from build123d import *

# Parameters (mm, degrees)
SKETCH1_W           = 22
SKETCH1_H           = 63.25
BOSS_EXTRUDE1_DEPTH = 17.4
SKETCH2_W           = 10.1
SKETCH2_H           = 7.15
CUT_EXTRUDE1_DEPTH  = 8.4
SKETCH3_R           = 2.325
CUT_EXTRUDE2_DEPTH  = 38.734607789


with BuildPart() as part:
    # Sketch1 → Boss-Extrude1 (new body)
    with BuildSketch(Plane(origin=(0, 0, 0), x_dir=(1, 0, 0), z_dir=(0, 1, 0))):
        Rectangle(SKETCH1_W, SKETCH1_H)
    extrude(amount=BOSS_EXTRUDE1_DEPTH)

    # Sketch2 → Cut-Extrude1 (cut)
    with BuildSketch(Plane(origin=(0, 17.4, 0), x_dir=(1, 0, 0), z_dir=(0, 1, 0))):
        with Locations((-5.95, 18.05)):
            Rectangle(SKETCH2_W, SKETCH2_H)
        with Locations((5.95, 18.05)):
            Rectangle(SKETCH2_W, SKETCH2_H)
        with Locations((-5.95, 9.025)):
            Rectangle(SKETCH2_W, SKETCH2_H)
        with Locations((5.95, 9.025)):
            Rectangle(SKETCH2_W, SKETCH2_H)
        with Locations((-5.95, 0)):
            Rectangle(SKETCH2_W, SKETCH2_H)
        with Locations((5.95, 0)):
            Rectangle(SKETCH2_W, SKETCH2_H)
        with Locations((-5.95, -9.025)):
            Rectangle(SKETCH2_W, SKETCH2_H)
        with Locations((5.95, -9.025)):
            Rectangle(SKETCH2_W, SKETCH2_H)
        with Locations((-5.95, -18.05)):
            Rectangle(SKETCH2_W, SKETCH2_H)
        with Locations((5.95, -18.05)):
            Rectangle(SKETCH2_W, SKETCH2_H)
    extrude(amount=-CUT_EXTRUDE1_DEPTH, mode=Mode.SUBTRACT)

    # Sketch3 → Cut-Extrude2 (cut, through all)
    with BuildSketch(Plane(origin=(0, 0, 0), x_dir=(1, 0, 0), z_dir=(0, 1, 0))):
        with Locations(Location((0, 26.675, 0), (0, 0, 270))):
            Circle(SKETCH3_R)
        with Locations(Location((0, -26.675, 0), (0, 0, 270))):
            Circle(SKETCH3_R)
    extrude(amount=CUT_EXTRUDE2_DEPTH, mode=Mode.SUBTRACT)


solid = part.part
Could you check a few things on this model? Use its own coordinates, in mm. A direction names the side the tool comes from. Coordinates: 2 decimals unless noted, no trailing zeros. Write each loop counter-clockwise with the first axis right and the second up, starting at its lowest first coordinate (ties: lowest second). Pieces come first, ordered by that corner, then holes. Notation, with made-up numbers: (46.5, -38.5) - (92.5, -38.5) arc R18 ccw to (92.5, -22.5) - close; hole circle Ø2 at (45.25, 1). An arc over 180 degrees is marked (long way). Put each result on its own line as item: value. Start each with the question number.
Q1. Which directions (+Z, -Z, +X, -X, +Y, -Y) give clear straight access to the entire face, cutting with the end or side of a thin tool? Please do faces 1 (the flat face through (0.9, 13, -9)), 2 (the cylindrical face through (0.698, 8.578, -24.457)), 3 (the flat face through (-0.9, 13, 0)).
Q2. Please list where these lines run through material, in increasing order: L1, parallel to Z at x = 0, y = 4.5 (3 decimals); L2, parallel to Z at x = -8.25, y = 15 (3 decimals); L3, parallel to Z at x = -0.5, y = 7.25 (3 decimals).
Q3. I want a section at D-D on y = 14.25. Count the separate pieces of the cut face and the enclosed holes in it, plus the area to 3 significant figures.
Q4. I'm going to push flat-ended pins straight in: P1, Ø2, axis at x = -5, z = 7.5, coming from the +Y side; P2, Ø4, axis at x = 0.5, z = 23.5, coming from the -Y side; P3, Ø2, axis at y = 14.5, z = 10.5, coming from the -X side. Where does each tip first touch, or does it pass through?
Q5. Thinking about a two-plate mould opening in Z: for faces 4 (the flat face through (11, 7, 0)), 5 (the flat face through (-0.9, 13, -18)), 6 (the cylindrical face through (1.57, 8.58, 24.96)), which applies, pulls with the +Z half, pulls with the -Z half, needs draft (parallel to the pull), parting line crosses it, or undercut?
Q6. I want a section at A-A on x = 0. Write out the boundary of the cut face in (y, z) (3 decimals).
Q7. I want a section at C-C on x = -3. Write out the boundary of the cut face in (y, z) (3 decimals), plus the area to 3 significant figures.
Q8. I want a section at B-B on z = -8. Write out the boundary of the cut face in (x, y), plus the area to 3 significant figures.
Checks:
1. face 1: +X, +Y
1. face 2: +Y, -Y
1. face 3: -X, +Y
2. L1: -31.625 to -29, -24.35 to 24.35, 29 to 31.625
2. L2: -31.625 to -21.625, -14.475 to -12.6, -5.45 to -3.575, 3.575 to 5.45, 12.6 to 14.475, 21.625 to 31.625
2. L3: -31.625 to -28.946, -24.404 to 24.404, 28.946 to 31.625
3. separate pieces: 1
3. enclosed holes: 2
3. area: 635 mm²
4. P1: y = 9
4. P2: y = 0
4. P3: x = -0.9
5. face 4: needs draft
5. face 5: undercut
5. face 6: undercut
6. outline: (0, -31.625) - (17.4, -31.625) - (17.4, -29) - (0, -29) - close; (0, -24.35) - (17.4, -24.35) - (17.4, 24.35) - (0, 24.35) - close; (0, 29) - (17.4, 29) - (17.4, 31.625) - (0, 31.625) - close
7. outline: (0, -31.625) - (17.4, -31.625) - (17.4, -21.625) - (9, -21.625) - (9, -14.475) - (17.4, -14.475) - (17.4, -12.6) - (9, -12.6) - (9, -5.45) - (17.4, -5.45) - (17.4, -3.575) - (9, -3.575) - (9, 3.575) - (17.4, 3.575) - (17.4, 5.45) - (9, 5.45) - (9, 12.6) - (17.4, 12.6) - (17.4, 14.475) - (9, 14.475) - (9, 21.625) - (17.4, 21.625) - (17.4, 31.625) - (0, 31.625) - close
7. area: 800 mm²
8. outline: (-11, 0) - (11, 0) - (11, 9) - (0.9, 9) - (0.9, 17.4) - (-0.9, 17.4) - (-0.9, 9) - (-11, 9) - close
8. area: 213 mm²
